Design review of the part shown in the three views and the two pictorial views. Dimensions are in mm from the part's minimum x, y and z. A direction names the side the tool comes from. Round coordinates to 2 decimals unless told otherwise and drop trailing zeros. Loops run counter-clockwise (first coordinate to the right, second up) from the corner with the lowest first, then second, coordinate; pieces in that order, holes last. Notation, with made-up numbers: (17, -19) - (74, -19) arc R21 ccw to (74, -6) - close; hole circle Ø4 at (16.25, 80). An arc over 180 degrees is marked (long way). Return JSON: item names as keys, results as strings. Group by question number.
(1) We need section B-B, the plane z = 5. Write out the cut boundary in (x, y), and give its area (3 significant figures).
(2) We need section A-A, the plane x = 21. Write out the cut boundary in (y, z), and give its area (3 significant figures).
(3) Clearance check with flat-ended pins moving along their axes: pin 1 (8 mm diameter, centred on y = 27.5, z = 12.5, fed in from +X); pin 2 (1.5 mm diameter, centred on x = 20.5, y = 30, fed in from +Z); pin 3 (2 mm diameter, centred on x = 21, y = 31, fed in from +Z). State where each tip first meets the part, or that it passes through.
(4) The part is to be moulded in two halves that separate along Y. For the marked faces 3, 4 and 5, say which applies: pulls with the +Y half, pulls with the -Y half, needs draft (parallel to the pull), parting line crosses it, or undercut.
(5) For the marked faces 1 and 2, list the 3-axis set-ups (+Z, -Z, +X, -X, +Y, -Y) from which the entire face can be reached by the end or side of a thin tool; tool diameter is ignored.
(6) Wall thickness on L1, parallel to Y at x = 21, z = 4.35; L2, parallel to Y at x = 21, z = 10; L3, parallel to Y at x = 21, z = 0.3: over which ranges is each line inside the solid? List them lowest first. Write a range as [from, to].
(7) We need section C-C, the plane z = 12.5. Write out the cut boundary in (x, y).
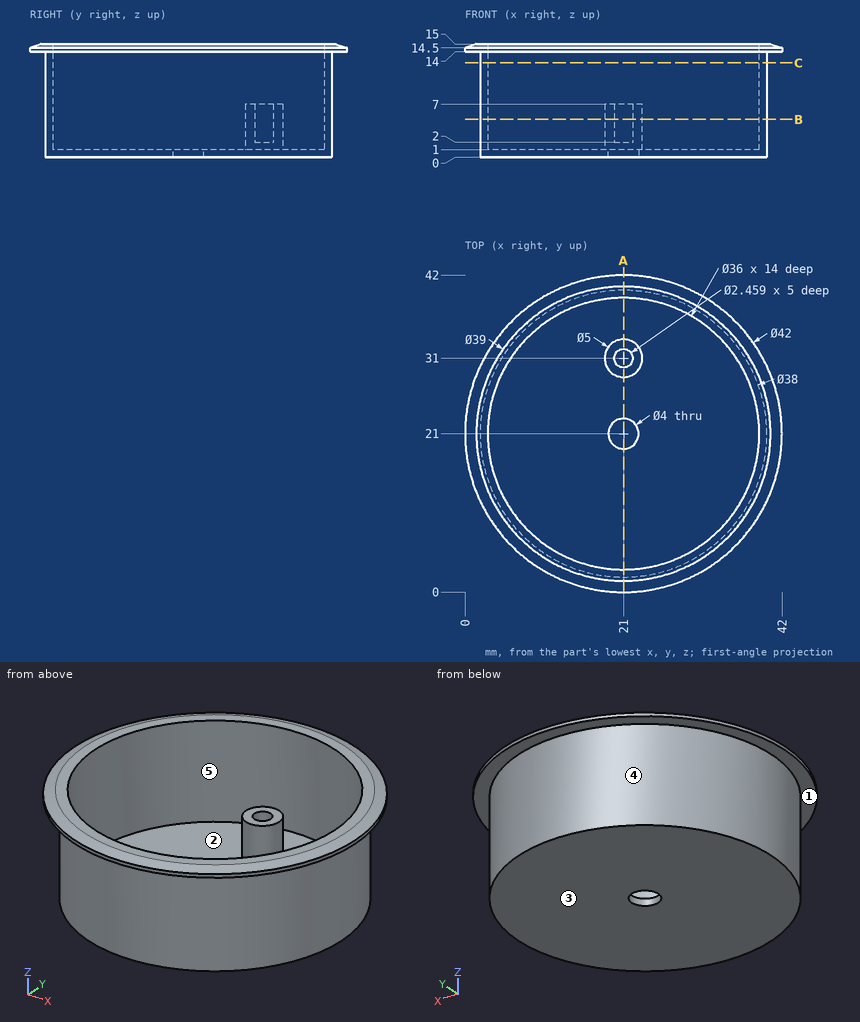
Solutions:
{
 "1": {"outline": "circle Ø38 at (21, 21); circle Ø5 at (21, 31); hole circle Ø36 at (21, 21); hole circle Ø2.46 at (21, 31)", "area": "131 mm^2"},
 "2": {"outline": "(0, 14) - (2, 14) - (2, 0) - (19, 0) - (19, 1) - (3, 1) - (3, 15) - (1.5, 15) - (0, 14.5) - close; (23, 0) - (40, 0) - (40, 14) - (42, 14) - (42, 14.5) - (40.5, 15) - (39, 15) - (39, 1) - (33.5, 1) - (33.5, 7) - (32.23, 7) - (32.23, 2) - (29.77, 2) - (29.77, 7) - (28.5, 7) - (28.5, 1) - (23, 1) - close", "area": "83.0 mm^2"},
 "3": {"pin 1": "x = 41.81", "pin 2": "z = 7", "pin 3": "z = 2"},
 "4": {"face 3": "needs draft", "face 4": "parting line crosses it", "face 5": "undercut"},
 "5": {"face 1": "-Z", "face 2": "+Z"},
 "6": {"L1": "[2, 3], [28.5, 29.77], [32.23, 33.5], [39, 40]", "L2": "[2, 3], [39, 40]", "L3": "[2, 19], [23, 40]"},
 "7": {"outline": "circle Ø38 at (21, 21); hole circle Ø36 at (21, 21)"}
}
